Check sheet for the modelled part. Datum: model origin and axes. Units: mm. Face numbers are marked on the shaded views. A direction names the side the tool comes from. Round coordinates to 2 decimals unless told otherwise and drop trailing zeros. Order: outer loops, then holes, each group sorted by start corner. A loop starts at its lowest first (then second) coordinate and runs counter-clockwise, first axis right, second up. Notation, with made-up numbers: M 35.25,-20.75 L 45.25,-20.75 A19 ccw 45.25,0.25 Z; hole C 24.25,-18 d11. An arc over 180 degrees is marked long. One line per item, written item: value. Start each with the question number.
(1) Cross-section at A-A, the plane y = -23.5. Enter the section's corners in (x, z), and give its area (3 significant figures).
(2) Access from +Z, -Z, +X, -X, +Y, -Y to the whole of each face (thin tool, end or side, straight path). Record for the marked faces 1, 2, 3, 4 and 5.
(3) Cross-section at C-C, the plane x = 14. Enter the section's corners in (y, z).
(4) Depth check by flat-ended pin: pin 1 Ø16.5 at (y, z) = (-25.1, -15) entering from +X; pin 2 Ø12 at (x, z) = (37, -24.5) entering from +Y; pin 3 Ø3 at (y, z) = (46.5, -25) entering from -X; pin 4 Ø7 at (y, z) = (-26, -14.5) entering from -X. Enter the tip coordinate at first touch or a pass-through.
(5) Cross-section at D-D, the plane y = 34. Enter the section's corners in (x, z).
(6) Release check for a two-part mould opening along Y. For the marked faces 6, 7 and 8 record: released by +Y, released by -Y, zero draft, split by the parting line, or undercut.
(7) Thickness scan on L1, parallel to X at y = -21, z = -6; L2, parallel to Z at x = 50, y = -20; L3, parallel to X at y = 23, z = -25. Record the ranges inside material, lowest first.
(8) Cross-section at B-B, the plane z = -15. Enter the section's corners in (x, y), and give its area (3 significant figures).
from build123d import *

# Parameters (mm, degrees)
SKETCH2_W           = 30
SKETCH2_H           = 100
EXTRUDE_THIN1_DEPTH = 60
CUT_EXTRUDE1_DEPTH  = 60
CUT_EXTRUDE2_DEPTH  = 60
CUT_EXTRUDE3_DEPTH  = 60
SKETCH6_R           = 6.257784416
CUT_EXTRUDE4_DEPTH  = 61
SKETCH7_R           = 3
CUT_EXTRUDE5_DEPTH  = 2
BOSS_EXTRUDE1_START = -75
SKETCH10_R          = 3
BOSS_EXTRUDE1_DEPTH = 90


with BuildPart() as part:
    # Sketch2 → Extrude-Thin1 (new body)
    with BuildSketch(Plane(origin=(0, 0, 0), x_dir=(0, 0, -1), z_dir=(1, 0, 0))):
        with Locations((15, 13.4875)):
            Rectangle(SKETCH2_W, SKETCH2_H)
    extrude(amount=EXTRUDE_THIN1_DEPTH)

    # Sketch3 → Cut-Extrude1 (cut)
    with BuildSketch(Plane(origin=(60, 0, 0), x_dir=(0, 0, -1), z_dir=(1, 0, 0))):
        Polygon((0, 63.4875), (0, -36.5125), (30, 63.4875), align=None)
    extrude(amount=-CUT_EXTRUDE1_DEPTH, mode=Mode.SUBTRACT)

    # Sketch4 → Cut-Extrude2 (cut)
    with BuildSketch(Plane(origin=(0, 0, -30), x_dir=(-1, 0, 0), z_dir=(0, 0, -1))):
        Polygon((-30, 63.4875), (-60, -13.684128909), (-60, 63.4875), align=None)
    extrude(amount=-CUT_EXTRUDE2_DEPTH, mode=Mode.SUBTRACT)

    # Sketch5 → Cut-Extrude3 (cut)
    with BuildSketch(Plane(origin=(0, 0, -30), x_dir=(-1, 0, 0), z_dir=(0, 0, -1))):
        Polygon((-30, 63.4875), (0, 63.4875), (0, -13.684128909), align=None)
    extrude(amount=-CUT_EXTRUDE3_DEPTH, mode=Mode.SUBTRACT)

    # Sketch6 → Cut-Extrude4 (cut, through all)
    with BuildSketch(Plane(origin=(60, 0, 0), x_dir=(0, 0, -1), z_dir=(1, 0, 0))):
        with Locations((15, -25.098314454)):
            Circle(SKETCH6_R)
    extrude(amount=-CUT_EXTRUDE4_DEPTH, mode=Mode.SUBTRACT)

    # Sketch7 → Cut-Extrude5 (cut)
    with BuildSketch(Plane(origin=(0, -3.014793578, -10.049311927), x_dir=(1, 0, 0), z_dir=(0, 0.287347886, 0.957826285))):
        with Locations((30, 55.48605385)):
            Circle(SKETCH7_R)
    extrude(amount=-CUT_EXTRUDE5_DEPTH, mode=Mode.SUBTRACT)

    # Sketch10 → Boss-Extrude1 (add)
    with BuildSketch(Plane(origin=(60, 0, 0), x_dir=(0, 0, -1), z_dir=(1, 0, 0)).offset(BOSS_EXTRUDE1_START)):
        with Locations((25.790784961, 6.968067419)):
            Circle(SKETCH10_R)
    extrude(amount=BOSS_EXTRUDE1_DEPTH)


solid = part.part
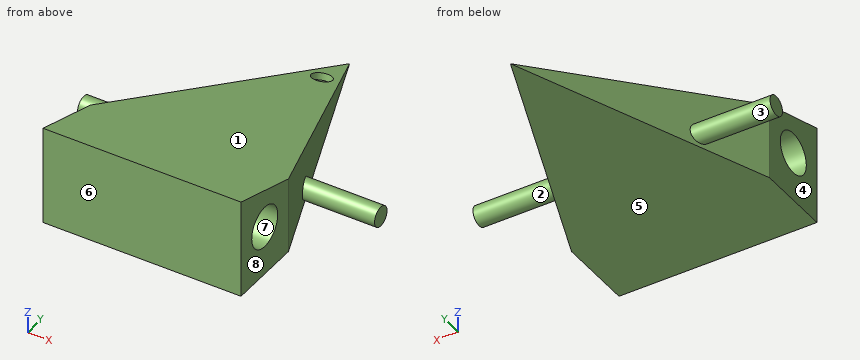
Values found:
1. outline: M 0,-30 L 60,-30 L 60,-21.05 L 0,-21.05 Z; M 0,-8.95 L 60,-8.95 L 60,-3.9 L 0,-3.9 Z
1. area: 840 mm^2
2. face 1: +Z, +X, -X, +Y
2. face 2: +X
2. face 3: -X
2. face 4: +Z, -Z, -X, -Y
2. face 5: -Z, +X, -X, +Y, -Y
3. outline: M -36.51,-30 L 22.33,-30 L 22.33,-17.65 L -36.51,0 Z; hole C -25.1,-15 d12.52
4. pin 1: x = 60
4. pin 2: y = 57.58
4. pin 3: x = 22.81
4. pin 4: through
5. outline: M 18.54,-30 L 41.46,-30 L 41.46,-21.15 L 18.54,-21.15 Z
6. face 6: released by -Y
6. face 7: undercut
6. face 8: zero draft
7. L1: 0 to 60
7. L2: -30 to -18.63, -11.37 to -4.95
7. L3: 14.26 to 45.74
8. outline: M 0,-36.51 L 60,-36.51 L 60,-31.36 L 0,-31.36 Z; M 0,-18.84 L 60,-18.84 L 60,-13.68 L 49.44,13.49 L 10.56,13.49 L 0,-13.68 Z
8. area: 1,960 mm^2
